Can you work these out from the model? Positions are in its coordinate system, mm. A direction names the side the tool comes from. Coordinates: 2 decimals unless noted, no trailing zeros. Order: outer loops, then holes, each group sorted by start corner. A loop starts at its lowest first (then second) coordinate and runs counter-clockwise, first axis right, second up. Notation, with made-up numbers: (-27, 12) - (19, 12) arc R21 cw to (19, 41) - close; hole circle Ø2 at (6, 49.25). An arc over 180 degrees is marked (long way). Use a Markdown table: item, result. Add a question column.
(1) For pin 1 Ø9 at (x, y) = (322, -37) entering from -Z; pin 2 Ø24 at (y, z) = (44, 29.5) entering from +X; pin 3 Ø20 at (x, y) = (291.5, 47) entering from -Z, each with a flat end and sliding along its axis, tell me the tip position at first contact or that it passes through.
(2) I want a section at B-B (z = 205). List the corners of the cut face in (x, y) for me, and give its area (3 significant figures).
(3) If I drill on L1, parallel to X at y = 37, z = 656.5; L2, parallel to Z at x = 291, y = 23.5; L3, parallel to X at y = 71.5, z = 57.5, over which ranges is the centre line in solid material (lowest first)? Write a range as [from, to].
(4) I want a section at A-A (y = -52). List the corners of the cut face in (x, z) for me.
(5) On a 3-axis mill with a long thin cutter (end or side, diameter ignored), from which of +Z, -Z, +X, -X, +Y, -Y can I reach the whole of each face in a straight line? I mean faces 1 (the flat face through (11, -100, 407)), 2 (the flat face through (275, -1, 41)). Say none if no direction works.
```python
from build123d import *

# Parameters (mm, degrees)
F0_W     = 600
F0_H     = 200
F1_DEPTH = 800
F2_W     = 200
F2_H     = 80
F3_DEPTH = 25
F4_W     = 630
F4_H     = 200
F5_DEPTH = 25


with BuildPart() as f1:
    # F0 (on Top) → F1 (new body)
    with BuildSketch(Plane.XY):
        Rectangle(F0_W, F0_H)
    extrude(amount=F1_DEPTH)

    # F2 (on face) → F3 (cut)
    with BuildSketch(Plane.YZ.offset(300)):
        with Locations((0, 40)):
            Rectangle(F2_W, F2_H)
    extrude(amount=-F3_DEPTH, mode=Mode.SUBTRACT)

    # F4 (on face) → F5 (join)
    with BuildSketch(Plane.XY.offset(800)):
        with Locations((15, 0)):
            Rectangle(F4_W, F4_H)
    extrude(amount=F5_DEPTH)


solid = f1.part
```
Answers follow:
| question | item | result |
|---|---|---|
| 1 | pin 1 | stops at z = 800 |
| 1 | pin 2 | stops at x = 275 |
| 1 | pin 3 | stops at z = 80 |
| 2 | outline | (-300, -100) - (300, -100) - (300, 100) - (-300, 100) - close |
| 2 | area | 120,000 mm² |
| 3 | L1 | x = [-300, 300] |
| 3 | L2 | z = [80, 825] |
| 3 | L3 | x = [-300, 275] |
| 4 | outline | (-300, 0) - (275, 0) - (275, 80) - (300, 80) - (300, 800) - (330, 800) - (330, 825) - (-300, 825) - close |
| 5 | face 1 | +Z, -Z, +X, -X, -Y |
| 5 | face 2 | -Z, +X, +Y, -Y |
